```python
from build123d import *

# Parameters (mm, degrees)
SKETCH1_R               = 1.2
BOSS_EXTRUDE1_DEPTH     = 15
SKETCH3_W               = 15
SKETCH3_H               = 36
BOSS_EXTRUDE3_DEPTH     = 1.5
BOSS_EXTRUDE4_DEPTH     = 19.5
SKETCH6_R               = 1.2
BOSS_EXTRUDE5_DEPTH     = 15
SKETCH7_W               = 2
SKETCH7_H               = 36
BOSS_EXTRUDE6_DEPTH     = 8
SKETCH8_W               = 6
SKETCH8_H               = 1
CUT_EXTRUDE1_DEPTH      = 5
SKETCH9_W               = 6
SKETCH9_H               = 1.5
CUT_EXTRUDE2_DEPTH      = 5
CUT_EXTRUDE3_DEPTH      = 94.234757467
CUT_EXTRUDE3_DEPTH_BACK = 94.234757467
SKETCH10_W              = 71.8
SKETCH10_H              = 8
SKETCH11_W              = 36
SKETCH11_H              = 10
CUT_EXTRUDE4_DEPTH      = 10
SKETCH12_W              = 15
SKETCH12_H              = 36
CUT_EXTRUDE5_DEPTH      = 10


with BuildPart() as part:
    # Sketch1 → Boss-Extrude1 (new body)
    with BuildSketch(Plane(origin=(0, 0, 0), x_dir=(1, 0, 0), z_dir=(0, 1, 0))):
        with BuildLine():
            Line((2.4, -23.4), (2.4, 23.4))
            ThreePointArc((2.4, 23.4), (2.107106781, 24.107106781), (1.4, 24.4))
            Line((1.4, 24.4), (-1.2, 24.4))
            ThreePointArc((-1.2, 24.4), (-2.614213562, 23.814213562), (-3.2, 22.4))
            Line((-3.2, 22.4), (-3.2, 20))
            Line((-3.2, 20), (-15, 20))
            Line((-15, 20), (-15, 18))
            Line((-15, 18), (0, 18))
            Line((0, 18), (0, -18))
            Line((0, -18), (-15, -18))
            Line((-15, -18), (-15, -20))
            Line((-15, -20), (-3.2, -20))
            Line((-3.2, -20), (-3.2, -22.4))
            ThreePointArc((-3.2, -22.4), (-2.614213562, -23.814213562), (-1.2, -24.4))
            Line((-1.2, -24.4), (1.4, -24.4))
            ThreePointArc((1.4, -24.4), (2.107106781, -24.107106781), (2.4, -23.4))
        make_face()
        with Locations(Location((0, -21.2, 0), (0, 0, 270))):
            Circle(SKETCH1_R, mode=Mode.SUBTRACT)
        with Locations(Location((0, 21.2, 0), (0, 0, 90))):
            Circle(SKETCH1_R, mode=Mode.SUBTRACT)
    extrude(amount=BOSS_EXTRUDE1_DEPTH)

    # Sketch3 → Boss-Extrude3 (add)
    with BuildSketch(Plane(origin=(0, 0, 0), x_dir=(1, 0, 0), z_dir=(0, 1, 0))):
        with Locations((-7.5, 0)):
            Rectangle(SKETCH3_W, SKETCH3_H)
    extrude(amount=BOSS_EXTRUDE3_DEPTH)

    # Sketch4 → Boss-Extrude4 (add)
    with BuildSketch(Plane.ZY.offset(15)):
        Polygon((-18, 1.5), (-18, 0), (-20, 0), (-20, 15), (-18, 15), align=None)
    extrude(amount=BOSS_EXTRUDE4_DEPTH)

    # Sketch6 → Boss-Extrude5 (add)
    # profile 1 of 2: a face of its own
    with BuildSketch(Plane(origin=(0, 15, 0), x_dir=(1, 0, 0), z_dir=(0, 1, 0))):
        with BuildLine():
            Line((-45.3, 20), (-45.3, 23.5))
            ThreePointArc((-45.3, 23.5), (-39.1, 29.7), (-32.9, 23.5))
            Line((-32.9, 23.5), (-32.9, 20))
            Line((-32.9, 20), (-34.5, 20))
            Line((-34.5, 20), (-34.5, 23.5))
            ThreePointArc((-34.5, 23.5), (-39.1, 28.1), (-43.7, 23.5))
            Line((-43.7, 23.5), (-43.7, 20))
            Line((-43.7, 20), (-43.7, 18))
            Line((-43.7, 18), (-80.6, 18))
            Line((-80.6, 18), (-80.6, 23.4))
            ThreePointArc((-80.6, 23.4), (-80.307106781, 24.107106781), (-79.6, 24.4))
            Line((-79.6, 24.4), (-77, 24.4))
            ThreePointArc((-77, 24.4), (-75.585786438, 23.814213562), (-75, 22.4))
            Line((-75, 22.4), (-75, 20))
            Line((-75, 20), (-45.3, 20))
        make_face()
        with Locations(Location((-78.2, 21.2, 0), (0, 0, 270))):
            Circle(SKETCH6_R, mode=Mode.SUBTRACT)
    # profile 2 of 2: a face of its own
    with BuildSketch(Plane(origin=(0, 15, 0), x_dir=(1, 0, 0), z_dir=(0, 1, 0))):
        with BuildLine():
            Line((-80.6, -18), (-15, -18))
            Line((-15, -18), (-15, -20))
            Line((-15, -20), (-75, -20))
            Line((-75, -20), (-75, -22.4))
            ThreePointArc((-75, -22.4), (-75.585786438, -23.814213562), (-77, -24.4))
            Line((-77, -24.4), (-79.6, -24.4))
            ThreePointArc((-79.6, -24.4), (-80.307106781, -24.107106781), (-80.6, -23.4))
            Line((-80.6, -23.4), (-80.6, -18))
        make_face()
        with Locations(Location((-78.2, -21.2, 0), (0, 0, 90))):
            Circle(SKETCH6_R, mode=Mode.SUBTRACT)
    extrude(amount=-BOSS_EXTRUDE5_DEPTH)

    # Sketch7 → Boss-Extrude6 (add)
    with BuildSketch(Plane.XZ):
        with Locations((-79.6, 0)):
            Rectangle(SKETCH7_W, SKETCH7_H)
    extrude(amount=-BOSS_EXTRUDE6_DEPTH)

    # Sketch8 → Cut-Extrude1 (cut)
    with BuildSketch(Plane(origin=(0, 0, 18), x_dir=(-1, 0, 0), z_dir=(0, 0, -1))):
        with Locations((39.1, 2)):
            Rectangle(SKETCH8_W, SKETCH8_H)
    extrude(amount=-CUT_EXTRUDE1_DEPTH, mode=Mode.SUBTRACT)

    # Sketch9 → Cut-Extrude2 (cut)
    with BuildSketch(Plane(origin=(-78.6, 0, 0), x_dir=(0, 0, -1), z_dir=(1, 0, 0))):
        with Locations((8, 3.25)):
            Rectangle(SKETCH9_W, SKETCH9_H)
        with Locations((-8, 3.25)):
            Rectangle(SKETCH9_W, SKETCH9_H)
    extrude(amount=-CUT_EXTRUDE2_DEPTH, mode=Mode.SUBTRACT)

    # Sketch10 → Cut-Extrude3 (cut, two sides: drawn at the far end of the back side and taken through both)
    with BuildSketch(Plane(origin=(0, 0, -20), x_dir=(-1, 0, 0), z_dir=(0, 0, -1)).offset(-CUT_EXTRUDE3_DEPTH_BACK)):
        with Locations((39.1, 11)):
            Rectangle(SKETCH10_W, SKETCH10_H)
    extrude(amount=CUT_EXTRUDE3_DEPTH + CUT_EXTRUDE3_DEPTH_BACK, mode=Mode.SUBTRACT)

    # Sketch11 → Cut-Extrude4 (cut)
    with BuildSketch(Plane(origin=(2.4, 0, 0), x_dir=(0, 0, -1), z_dir=(1, 0, 0))):
        with Locations((0, 10)):
            Rectangle(SKETCH11_W, SKETCH11_H)
    extrude(amount=-CUT_EXTRUDE4_DEPTH, mode=Mode.SUBTRACT)

    # Sketch12 → Cut-Extrude5 (cut)
    with BuildSketch(Plane.XZ):
        with Locations((-7.5, 0)):
            Rectangle(SKETCH12_W, SKETCH12_H)
    extrude(amount=-CUT_EXTRUDE5_DEPTH, mode=Mode.SUBTRACT)


solid = part.part
```
Check sheet for the modelled part. Datum: model origin and axes. Units: mm. A direction names the side the tool comes from. Give positions to 0.01 mm unless a question says otherwise; leave off trailing zeros. Order: outer loops, then holes, each group sorted by start corner. A loop starts at its lowest first (then second) coordinate and runs counter-clockwise, first axis right, second up. Notation, with made-up numbers: M 63.5,-24 L 72.5,-24 A31 cw 72.5,7 Z; hole C 41.25,59.25 d10. An arc over 180 degrees is marked long. Answer in a Markdown table with one row per item. Add a question column.
Q1. Sectioned sample at B-B, the plane z = -8. Record the boundary of the cut face in (x, y), and give its area (3 significant figures).
Q2. Gauge pin test, flat ends, axial feed: pin 1 Ø5 at (y, z) = (12.5, 1) entering from +X; pin 2 Ø8 at (y, z) = (9.5, -8.5) entering from +X; pin 3 Ø8 at (y, z) = (11, -13.5) entering from -X; pin 4 Ø1.2 at (x, y) = (-79.5, 3.5) entering from -Z. Record the tip position at first contact, or that the pin passes through.
Q3. Sectioned sample at A-A, the plane y = 13.5. Record the boundary of the cut face in (x, z), and give its area (3 significant figures).
Q4. Thickness scan on L1, parallel to X at y = 9.25, z = 21.2; L2, parallel to Z at x = -78.2, y = 10.75; L3, parallel to X at y = 4.25, z = -21.2. Record the ranges inside material, lowest first.
Q5. Sectioned sample at D-D, the plane z = -21.2. Record the boundary of the cut face in (x, y).
Q6. Sectioned sample at C-C, the plane x = -10.5. Record the boundary of the cut face in (y, z).
Q7. Access from +Z, -Z, +X, -X, +Y, -Y to the whole of each face (thin tool, end or side, straight path). Record for faces 1 (the flat face through (-60, 4, -20)), 2 (the flat face through (-34.5, 4, -21)), 3 (the flat face through (-78, 8, -24.4)).
Q8. Release check for a two-part mould opening along X. For faces 4 (the flat face through (-18, 3, -20)), 5 (the cylindrical face through (0.36, 7.395, 22.345)), 6 (the flat face through (-80, 2.5, 8)) record: released by +X, released by -X, zero draft, split by the parting line, or undercut.
Verdict:
| question | item | result |
|---|---|---|
| 1 | outline | M -80.6,0 L -78.6,0 L -78.6,2.5 L -80.6,2.5 Z; M -80.6,4 L -78.6,4 L -78.6,8 L -80.6,8 Z; M 0,0 L 2.4,0 L 2.4,5 L 0,5 Z |
| 1 | area | 25.0 mm² |
| 2 | pin 1 | through |
| 2 | pin 2 | x = -78.6 |
| 2 | pin 3 | x = -80.6 |
| 2 | pin 4 | z = -24.4 |
| 3 | outline | M -80.6,-23.4 A1 ccw -79.6,-24.4 L -77,-24.4 A2 ccw -75,-22.4 L -75,-18 L -80.6,-18 Z; M -80.6,18 L -75,18 L -75,22.4 A2 ccw -77,24.4 L -79.6,24.4 A1 ccw -80.6,23.4 Z; M -3.2,-22.4 A2 ccw -1.2,-24.4 L 1.4,-24.4 A1 ccw 2.4,-23.4 L 2.4,-18 L -3.2,-18 Z; M -3.2,18 L 2.4,18 L 2.4,23.4 A1 ccw 1.4,24.4 L -1.2,24.4 A2 ccw -3.2,22.4 Z; hole C -78.2,-21.2 d2.4; hole C -78.2,21.2 d2.4; hole C 0,-21.2 d2.4; hole C 0,21.2 d2.4 |
| 3 | area | 121 mm² |
| 4 | L1 | -80.6 to -79.4, -77 to -75, -3.2 to -1.2, 1.2 to 2.4 |
| 4 | L2 | -24.4 to -22.4, -20 to -18, 18 to 20, 22.4 to 24.4 |
| 4 | L3 | -80.6 to -79.4, -77 to -75, -45.3 to -43.7, -34.5 to -32.9, -3.2 to -1.2, 1.2 to 2.4 |
| 5 | outline | M -80.6,0 L -79.4,0 L -79.4,15 L -80.6,15 Z; M -77,0 L -75,0 L -75,15 L -77,15 Z; M -45.3,0 L -43.7,0 L -43.7,7 L -45.3,7 Z; M -34.5,0 L -32.9,0 L -32.9,7 L -34.5,7 Z; M -3.2,0 L -1.2,0 L -1.2,15 L -3.2,15 Z; M 1.2,0 L 2.4,0 L 2.4,15 L 1.2,15 Z |
| 6 | outline | M 0,-20 L 7,-20 L 7,-18 L 0,-18 Z; M 0,18 L 7,18 L 7,20 L 0,20 Z |
| 7 | face 1 | -Z, +Y, -Y |
| 7 | face 2 | +Y, -Y |
| 7 | face 3 | -Z, -X, +Y, -Y |
| 8 | face 4 | undercut |
| 8 | face 5 | undercut |
| 8 | face 6 | zero draft |
